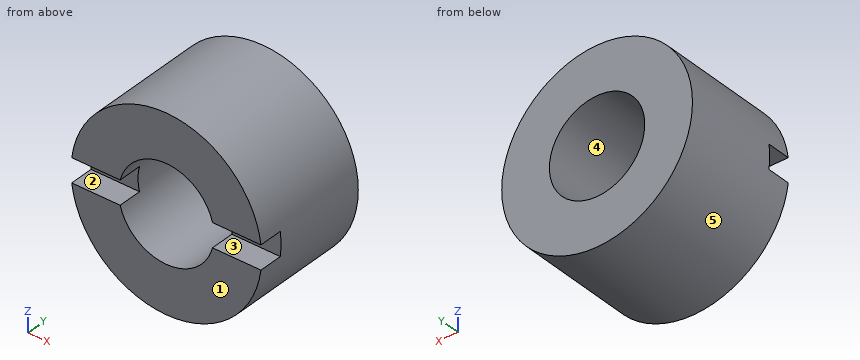
```python
from build123d import *

# Parameters (mm, degrees)
SKETCH2_W               = 4
SKETCH2_H               = 10
SKETCH3_W               = 2
SKETCH3_H               = 2
CUT_EXTRUDE1_DEPTH      = 9
CUT_EXTRUDE1_DEPTH_BACK = 9


with BuildPart() as part:
    # Sketch2 → Revolve1 (revolve)
    with BuildSketch(Plane(origin=(0, 0, 0), x_dir=(0, 0, -1), z_dir=(1, 0, 0))):
        with Locations((6, -0.173076923)):
            Rectangle(SKETCH2_W, SKETCH2_H)
    revolve(axis=Axis((0, 8.057692308, 0), (0, -1, 0)))

    # Sketch3 → Cut-Extrude1 (cut, two sides)
    with BuildSketch(Plane(origin=(0, 0, 0), x_dir=(0, 0, -1), z_dir=(1, 0, 0))) as cut_extrude1_sk:
        with Locations((0, -4.173076923)):
            Rectangle(SKETCH3_W, SKETCH3_H)
    extrude(amount=CUT_EXTRUDE1_DEPTH, mode=Mode.SUBTRACT)
    extrude(cut_extrude1_sk.sketch, amount=-CUT_EXTRUDE1_DEPTH_BACK, mode=Mode.SUBTRACT)


solid = part.part
```
CAD build for the part. Positions are in the model's coordinates, mm. Face numbers are marked on the shaded views. A direction names the side the tool comes from. Coordinates: 2 decimals unless noted, no trailing zeros. Write each loop counter-clockwise with the first axis right and the second up, starting at its lowest first coordinate (ties: lowest second). Pieces come first, ordered by that corner, then holes.
(1) Drill centre lines: probe 1 along X at (y, z) = (0.5, 0); probe 2 along X at (y, z) = (-2.75, -1). Where is each one in solid material? Low to high.
(2) Cut at A-A, the plane x = 0. List the corners of the cut face in (y, z), and give its area (3 significant figures).
(3) Cut at B-B, the plane z = 0. List the corners of the cut face in (x, y).
(4) Cut at D-D, the plane x = 5.75. List the corners of the cut face in (y, z).
(5) 3-axis set-ups, long thin cutter, end or side, ignore diameter. For the marked faces 1 and 2: which of +Z, -Z, +X, -X, +Y, -Y reach the whole face in a straight line?
(6) Cut at C-C, the plane y = -1.25. List the corners of the cut face in (x, z), and give its area (3 significant figures).
(7) Flat gauge pins, fed straight in: pin 1 (2 mm diameter, centred on x = -6, y = -4.5, fed in from +Z) (3 decimals); pin 2 (2 mm diameter, centred on x = 5.5, y = -4.5, fed in from +Z); pin 3 (3 mm diameter, centred on x = -1.5, y = -1.5, fed in from +Z); pin 4 (2 mm diameter, centred on x = -6.5, y = -4, fed in from -Z). Where does each tip first touch, or does it go through?
(8) Two-plate mould, pull along X, no slides. Class the marked faces 3, 4 and 5: +X half, -X half, draft (parallel to the pull), parting line (faces both ways), or undercut.
Geometry says:
1. probe 1: x = -8 to -4, 4 to 8
1. probe 2: x = -7.94 to -3.87, 3.87 to 7.94
2. outline: (-5.17, -8) - (4.83, -8) - (4.83, -4) - (-5.17, -4) - close; (-5.17, 4) - (4.83, 4) - (4.83, 8) - (-5.17, 8) - close
2. area: 80.0 mm2
3. outline: (-8, -3.17) - (-4, -3.17) - (-4, 4.83) - (-8, 4.83) - close; (4, -3.17) - (8, -3.17) - (8, 4.83) - (4, 4.83) - close
4. outline: (-5.17, -5.56) - (4.83, -5.56) - (4.83, 5.56) - (-5.17, 5.56) - (-5.17, 1) - (-3.17, 1) - (-3.17, -1) - (-5.17, -1) - close
5. face 1: +Z, -Z, +X, -X, -Y
5. face 2: +X, -X, -Y
6. outline: circle Ø16 at (0, 0); hole circle Ø8 at (0, 0)
6. area: 151 mm2
7. pin 1: stops at z = 6.245
7. pin 2: stops at z = 6.61
7. pin 3: stops at z = 8
7. pin 4: stops at z = -5.81
8. face 3: draft
8. face 4: undercut
8. face 5: parting line
